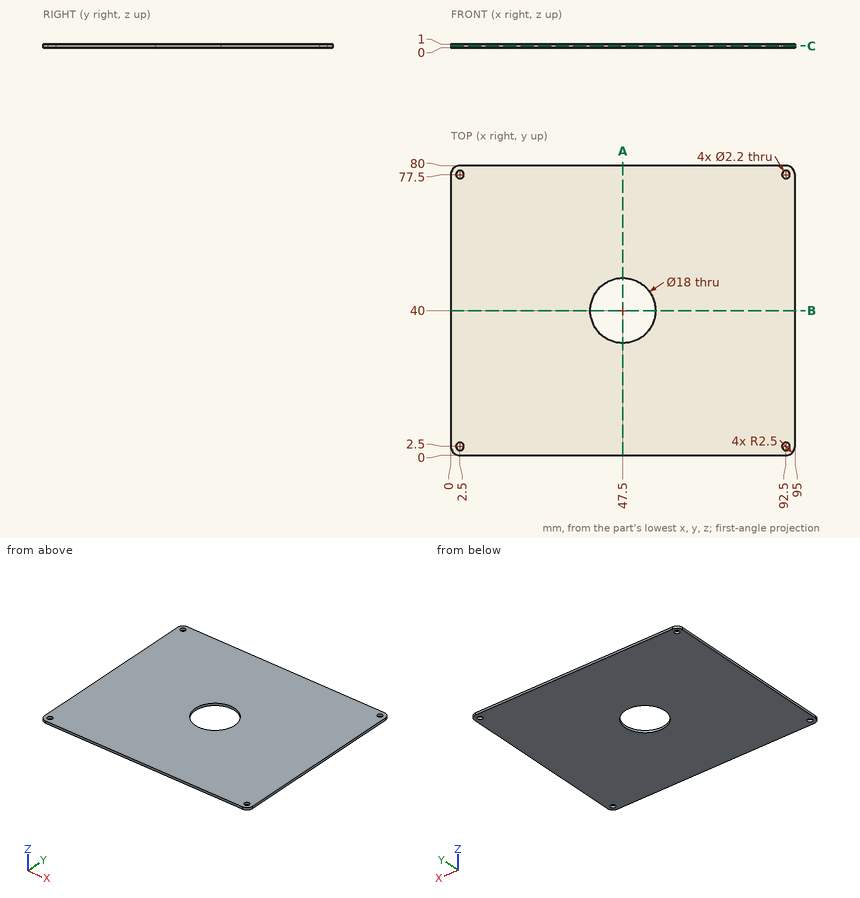
The figure shows three views and two pictorial views of one solid part (mm, origin at its lowest corner). Answer the questions. Give positions to 0.01 mm unless a question says otherwise; leave off trailing zeros. Order: outer loops, then holes, each group sorted by start corner. A loop starts at its lowest first (then second) coordinate and runs counter-clockwise, first axis right, second up. Notation, with made-up numbers: (53, 88) -> (92, 88) arc R22 cw to (92, 106) -> close; hole circle Ø10 at (66.25, 47.5). An arc over 180 degrees is marked (long way). Answer as a JSON object with one key per item and string values. Group by question number.
Item 1: The part is cut by section C-C on z = 0.45. Write down the section's boundary in (x, y), and give its area (3 significant figures).
Item 2: The part is cut by section B-B on y = 40. Write down the section's boundary in (x, z).
Item 3: The part is cut by section A-A on x = 47.5. Write down the section's boundary in (y, z), and give its area (3 significant figures).
Item 4: Consider L1, parallel to X at y = 2.5, z = 0.55; L2, parallel to X at y = 44, z = 0.75; L3, parallel to Y at x = 51.5, z = 0.2. Determine where each line is inside the solid, lowest interval first. Write a range as from..to.
Result set:
{
 "1": {"outline": "(0, 2.5) arc R2.5 ccw to (2.5, 0) -> (92.5, 0) arc R2.5 ccw to (95, 2.5) -> (95, 77.5) arc R2.5 ccw to (92.5, 80) -> (2.5, 80) arc R2.5 ccw to (0, 77.5) -> close; hole circle Ø2.2 at (2.5, 2.5); hole circle Ø2.2 at (2.5, 77.5); hole circle Ø18 at (47.5, 40); hole circle Ø2.2 at (92.5, 2.5); hole circle Ø2.2 at (92.5, 77.5)", "area": "7,320 mm²"},
 "2": {"outline": "(0, 0) -> (38.5, 0) -> (38.5, 1) -> (0, 1) -> close; (56.5, 0) -> (95, 0) -> (95, 1) -> (56.5, 1) -> close"},
 "3": {"outline": "(0, 0) -> (31, 0) -> (31, 1) -> (0, 1) -> close; (49, 0) -> (80, 0) -> (80, 1) -> (49, 1) -> close", "area": "62.0 mm²"},
 "4": {"L1": "0..1.4, 3.6..91.4, 93.6..95", "L2": "0..39.44, 55.56..95", "L3": "0..31.94, 48.06..80"}
}
